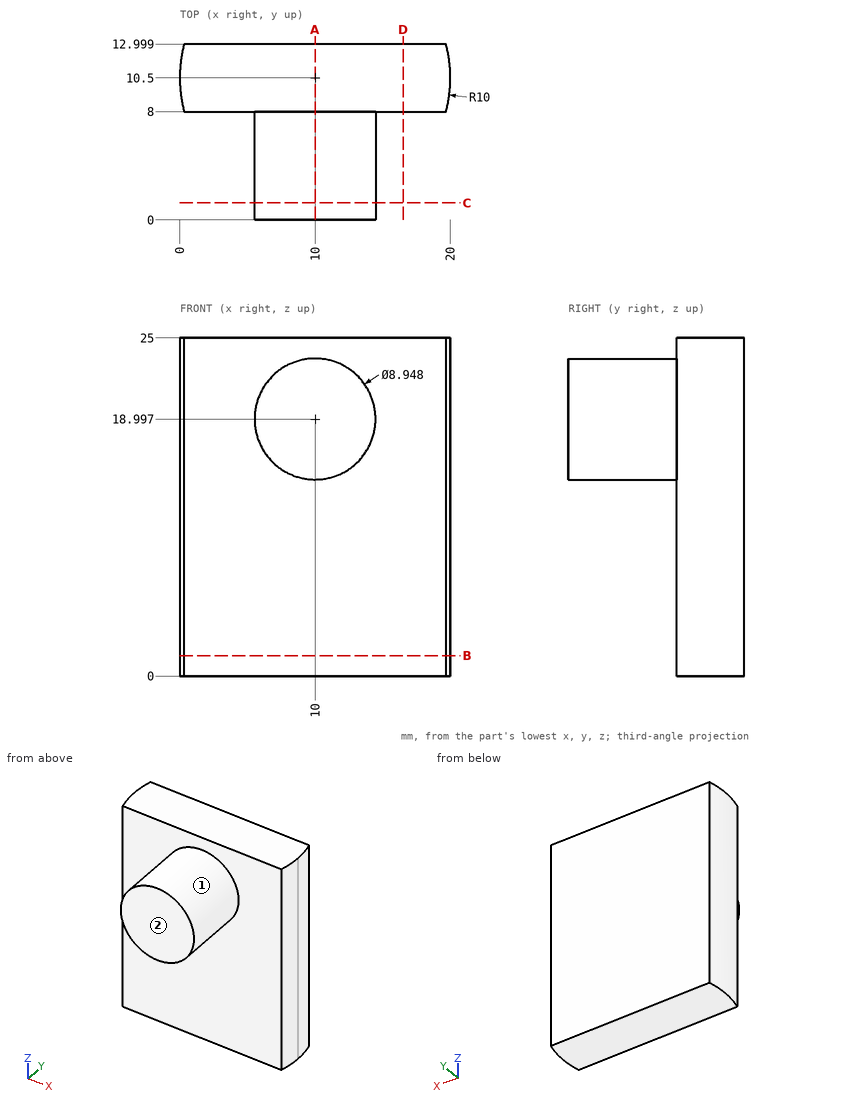
Verification items for this drawing (mm, ordinates from the low corner). A direction names the side the tool comes from. Coordinates: 2 decimals unless noted, no trailing zeros. Order: outer loops, then holes, each group sorted by start corner. A loop starts at its lowest first (then second) coordinate and runs counter-clockwise, first axis right, second up. Notation, with made-up numbers: (-27.5, 80.5) -> (20.5, 80.5) arc R22 ccw to (20.5, 94.5) -> close; hole circle Ø5 at (27, 51). An arc over 180 degrees is marked (long way). Answer as CSV lines item,"result". Start each with the question number.
1) Material ranges on L1, parallel to Y at x = 16.25, z = 3.5; L2, parallel to Z at x = 12.75, y = 6 (1 decimal); L3, parallel to Z at x = 9.5, y = 7, recorded low to high. Write a range as [from, to].
2) Gauge pin test, flat ends, axial feed: pin 1 Ø3 at (y, z) = (8.5, 13) entering from -X; pin 2 Ø9.5 at (x, z) = (11, 9.5) entering from -Y. Record the tip position at first contact, or that the pin passes through.
3) Cross-section at D-D, the plane x = 16.5. Record the boundary of the cut face in (y, z).
4) Set-up check for the marked faces 1 and 2: record each of +Z, -Z, +X, -X, +Y, -Y from which the full face is reachable in a straight line by a thin tool's end or side.
5) Cross-section at C-C, the plane y = 1.25. Record the boundary of the cut face in (x, z).
6) Cross-section at A-A, the plane x = 10. Record the boundary of the cut face in (y, z).
7) Cross-section at B-B, the plane z = 1.5. Record the boundary of the cut face in (x, y).
Conclusion:
1,L1,"y = [8, 13]"
1,L2,"z = [15.5, 22.5]"
1,L3,"z = [14.55, 23.44]"
2,pin 1,"stops at x = 0.01"
2,pin 2,"stops at y = 8"
3,outline,"(8, 0) -> (13, 0) -> (13, 25) -> (8, 25) -> close"
4,face 1,"-Y"
4,face 2,"+Z, -Z, +X, -X, -Y"
5,outline,"circle Ø8.95 at (10, 19)"
6,outline,"(0, 14.52) -> (8, 14.52) -> (8, 0) -> (13, 0) -> (13, 25) -> (8, 25) -> (8, 23.47) -> (0, 23.47) -> close"
7,outline,"(0.32, 8) -> (19.68, 8) arc R10 ccw to (20, 10.5) arc R10 ccw to (19.68, 13) -> (0.32, 13) arc R10 ccw to start"
